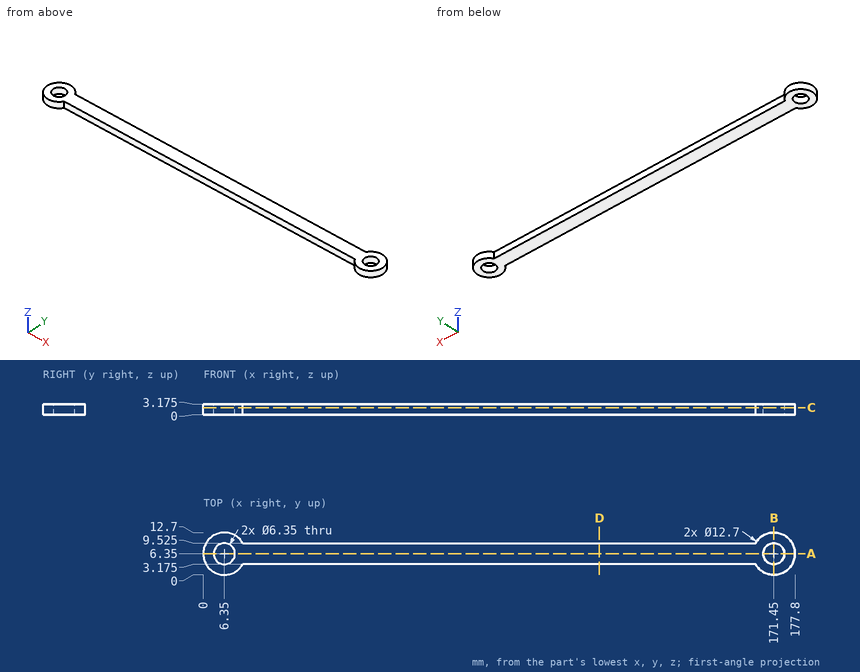
Verification items for this drawing (mm, ordinates from the low corner). Round coordinates to 2 decimals unless told otherwise and drop trailing zeros. Loops run counter-clockwise (first coordinate to the right, second up) from the corner with the lowest first, then second, coordinate; pieces in that order, holes last. Notation, with made-up numbers: M 35,55.25 L 91,55.25 A24 cw 91,71.25 Z; hole C 64,58 d5. An arc over 180 degrees is marked long. Answer as a JSON object with one key per item and string values.
1. Scan lines: line 1 (X direction, y = 6.25, z = 1.8); line 2 (X direction, y = 9.25, z = 1.65); line 3 (X direction, y = 2.5, z = 2.25). Record each from-to range of solid material in increasing order.
Reply:
{"line 1": "x = 0 to 3.18, 9.52 to 168.28, 174.62 to 177.8", "line 2": "x = 0.7 to 5.06, 7.64 to 170.16, 172.74 to 177.1", "line 3": "x = 1.3 to 11.4, 166.4 to 176.5"}
2. Section check A-A (y = 6.35). Record the boundary of the cut face in (x, z) (3 decimals), plus the area to 3 significant figures.
Reply:
{"outline": "M 0,0 L 3.175,0 L 3.175,3.175 L 0,3.175 Z; M 9.525,0 L 168.275,0 L 168.275,3.175 L 9.525,3.175 Z; M 174.625,0 L 177.8,0 L 177.8,3.175 L 174.625,3.175 Z", "area": "524 mm²"}
3. Section check C-C (z = 2.1). Record the boundary of the cut face in (x, y) (3 decimals), plus the area to 3 significant figures.
Reply:
{"outline": "M 11.849,3.175 L 165.951,3.175 A6.35 ccw long 165.951,9.525 L 11.849,9.525 A6.35 ccw long Z; hole C 6.35,6.35 d6.35; hole C 171.45,6.35 d6.35", "area": "1,160 mm²"}
4. Section check D-D (x = 119). Record the boundary of the cut face in (y, z) (3 decimals), plus the area to 3 significant figures.
Reply:
{"outline": "M 3.175,0 L 9.525,0 L 9.525,3.175 L 3.175,3.175 Z", "area": "20.2 mm²"}
5. Section check B-B (x = 171.45). Record the boundary of the cut face in (y, z) (3 decimals), plus the area to 3 significant figures.
Reply:
{"outline": "M 0,0 L 3.175,0 L 3.175,3.175 L 0,3.175 Z; M 9.525,0 L 12.7,0 L 12.7,3.175 L 9.525,3.175 Z", "area": "20.2 mm²"}
6. Gauge pin test, flat end, axial feed: P1, Ø1.5, axis at x = 156.5, z = 0.5, coming from the -Y side (3 decimals). Record the tip position at first contact, or that the pin passes through.
Reply:
{"P1": "stops at y = 3.175"}
